Model file for the job. Use its own axes, mm. A direction names the side the tool comes from. Round coordinates to 2 decimals unless told otherwise and drop trailing zeros. Write each loop counter-clockwise with the first axis right and the second up, starting at its lowest first coordinate (ties: lowest second). Pieces come first, ordered by that corner, then holes. Notation, with made-up numbers: (11, 54) - (56, 54) arc R21 cw to (56, 62) - close; hole circle Ø9 at (3, 46). An arc over 180 degrees is marked (long way). Answer as a JSON object with one key per item and string values. Group by question number.
from build123d import *

# Parameters (mm, degrees)
BOSS_EXTRUDE1_DEPTH     = 14.5
CUT_EXTRUDE2_DEPTH      = 32.662280398
CUT_EXTRUDE2_DEPTH_BACK = 32.662280398
SKETCH4_R               = 1.1
SKETCH4_W               = 11
SKETCH4_H               = 11
SKETCH5_R               = 1.25
SKETCH5_R_2             = 1.6
CUT_EXTRUDE3_DEPTH      = 32.662280398
FILLET1_R               = 3


with BuildPart() as part:
    # Sketch1 → Boss-Extrude1 (new, symmetric)
    with BuildSketch(Plane(origin=(0, 0, 0), x_dir=(1, 0, 0), z_dir=(0, 1, 0))):
        Polygon((-7.131727984, 0), (-27.5, 0), (-27.5, -4), (-12.5, -4), (-12.5, -10), (12.5, -10), (12.5, -4), (27.5, -4), (27.5, 0), (7.131727984, 0), (0, -7.131727984), align=None)
    extrude(amount=BOSS_EXTRUDE1_DEPTH, both=True)

    # Sketch4 → Cut-Extrude2 (cut, two sides: drawn at the far end of the back side and taken through both)
    with BuildSketch(Plane.XY.offset(4).offset(-CUT_EXTRUDE2_DEPTH_BACK)):
        with Locations((22.5, 10)):
            Circle(SKETCH4_R)
        with Locations((22.5, -10)):
            Circle(SKETCH4_R)
        with Locations((22, 0)):
            Rectangle(SKETCH4_W, SKETCH4_H)
    extrude(amount=CUT_EXTRUDE2_DEPTH + CUT_EXTRUDE2_DEPTH_BACK, mode=Mode.SUBTRACT)

    # Sketch5 → Cut-Extrude3 (cut, through all)
    with BuildSketch(Plane.XY.offset(4)):
        with Locations((-22.5, 10)):
            Circle(SKETCH5_R)
        with Locations((-22.5, -10)):
            Circle(SKETCH5_R_2)
    extrude(amount=-CUT_EXTRUDE3_DEPTH, mode=Mode.SUBTRACT)

    # Fillet1
    fillet1_edges = [part.edges().sort_by_distance(p)[0] for p in [
        (-12.5, 0, 4),
        (12.5, 0, 4),
    ]]
    fillet(fillet1_edges, radius=FILLET1_R)


solid = part.part
(1) Slice it at D-D (z = 5). Write the cut outline in (x, y), then the cut area to 3 significant figures.
(2) Pull direction X, two halves, no side cores. Call faces 1 (the cylindrical face through (21.4, -10, 2)), 2 (the flat face through (27.5, 10, 2)), 3 (the flat face through (-0.4, -14.5, 7.2)): pulls with the +X half, pulls with the -X half, needs draft (parallel to the pull), parting line crosses it, or undercut.
(3) Slice it at A-A (x = -22.5). Write the cut outline in (y, z), then the cut area to 3 significant figures.
(4) Slice it at B-B (y = 10). Write the cut outline in (x, z), then the cut area to 3 significant figures.
(5) Flat gauge pins, fed straight in: pin 1 (2 mm diameter, centred on y = 2, z = 1.5, fed in from +X); pin 2 (13 mm diameter, centred on x = 20, y = -6, fed in from +Z); pin 3 (2.5 mm diameter, centred on x = 22.5, y = -10, fed in from +Z). Where does each tip first touch, or does it go through?
(6) Slice it at C-C (z = 1.75). Write the cut outline in (x, y).
(7) Drill centre lines: line 1 (Y direction, x = 22.5, z = 1.1); line 2 (Y direction, x = 19, z = 2); line 3 (X direction, y = 12, z = 3.5). Where is each one in solid material? Low to high. Write a range as from..to.
(8) 3-axis set-ups, long thin cutter, end or side, ignore diameter. For faces 4 (the flat face through (-3.516, 0.203, 3.616)), 5 (the flat face through (-12.5, 0, 8)), 6 (the flat face through (22, 5.5, 2)): which of +Z, -Z, +X, -X, +Y, -Y reach the whole face in a straight line?
Answer:
{
 "1": {"outline": "(-13.26, -14.5) - (-2.13, -14.5) - (-2.13, 14.5) - (-13.26, 14.5) - close; (2.13, -14.5) - (13.26, -14.5) - (13.26, 14.5) - (2.13, 14.5) - close", "area": "646 mm²"},
 "2": {"face 1": "undercut", "face 2": "pulls with the +X half", "face 3": "needs draft"},
 "3": {"outline": "(-14.5, 0) - (-11.6, 0) - (-11.6, 4) - (-14.5, 4) - close; (-8.4, 0) - (8.75, 0) - (8.75, 4) - (-8.4, 4) - close; (11.25, 0) - (14.5, 0) - (14.5, 4) - (11.25, 4) - close", "area": "93.2 mm²"},
 "4": {"outline": "(-27.5, 0) - (-23.75, 0) - (-23.75, 4) - (-27.5, 4) - close; (-21.25, 0) - (-7.13, 0) - (0, 7.13) - (7.13, 0) - (21.4, 0) - (21.4, 4) - (15.5, 4) arc R3 cw to (12.5, 7) - (12.5, 10) - (-12.5, 10) - (-12.5, 7) arc R3 cw to (-15.5, 4) - (-21.25, 4) - close; (23.6, 0) - (27.5, 0) - (27.5, 4) - (23.6, 4) - close", "area": "304 mm²"},
 "5": {"pin 1": "x = 16.5", "pin 2": "z = 4.76", "pin 3": "z = 4"},
 "6": {"outline": "(-27.5, -14.5) - (-5.38, -14.5) - (-5.38, 14.5) - (-27.5, 14.5) - close; (5.38, -14.5) - (27.5, -14.5) - (27.5, -5.5) - (16.5, -5.5) - (16.5, 5.5) - (27.5, 5.5) - (27.5, 14.5) - (5.38, 14.5) - close; hole circle Ø3.2 at (-22.5, -10); hole circle Ø2.5 at (-22.5, 10); hole circle Ø2.2 at (22.5, -10); hole circle Ø2.2 at (22.5, 10)"},
 "7": {"line 1": "-14.5..-11.1, -8.9..-5.5, 5.5..8.9, 11.1..14.5", "line 2": "-14.5..-5.5, 5.5..14.5", "line 3": "-27.5..-3.63, 3.63..27.5"},
 "8": {"face 4": "-Z, +Y, -Y", "face 5": "+Z, -X, +Y, -Y", "face 6": "+Z, -Z, +X"}
}
